```python
from build123d import *

# Parameters (mm, degrees)
SKETCH_1_R      = 50
EXTRUDE_1_DEPTH = 10


with BuildPart() as part:
    # ｽｹｯﾁ1 → ﾎﾞｽ - 押し出し1 (new body)
    with BuildSketch(Plane(origin=(0, 0, 0), x_dir=(1, 0, 0), z_dir=(0, 1, 0))):
        Circle(SKETCH_1_R)
        with BuildLine():
            Line((-3.420201433, 9.396926208), (-13.680805733, 37.587704831))
            ThreePointArc((-13.680805733, 37.587704831), (0, 40), (13.680805733, 37.587704831))
            Line((13.680805733, 37.587704831), (3.420201433, 9.396926208))
            ThreePointArc((3.420201433, 9.396926208), (0, 10), (-3.420201433, 9.396926208))
        make_face(mode=Mode.SUBTRACT)
        with BuildLine():
            Line((6.428376097, 7.661310457), (25.712004387, 30.64264375))
            ThreePointArc((25.712004387, 30.64264375), (34.641516151, 20.000866025), (39.39281012, 6.946793132))
            Line((39.39281012, 6.946793132), (9.84857753, 1.737347802))
            ThreePointArc((9.84857753, 1.737347802), (8.660754038, 5.000866025), (6.428376097, 7.661310457))
        make_face(mode=Mode.SUBTRACT)
        with BuildLine():
            Line((9.84957753, -1.735615751), (39.39381012, -6.945061081))
            ThreePointArc((39.39381012, -6.945061081), (34.642516151, -19.999133975), (25.713004387, -30.640911699))
            Line((25.713004387, -30.640911699), (6.429376097, -7.659578406))
            ThreePointArc((6.429376097, -7.659578406), (8.661754038, -4.999133975), (9.84957753, -1.735615751))
        make_face(mode=Mode.SUBTRACT)
        with BuildLine():
            Line((3.422201433, -9.396926208), (13.682805733, -37.587704831))
            ThreePointArc((13.682805733, -37.587704831), (0.002, -40), (-13.678805733, -37.587704831))
            Line((-13.678805733, -37.587704831), (-3.418201433, -9.396926208))
            ThreePointArc((-3.418201433, -9.396926208), (0.002, -10), (3.422201433, -9.396926208))
        make_face(mode=Mode.SUBTRACT)
        with BuildLine():
            Line((-6.426376097, -7.661310457), (-25.710004387, -30.64264375))
            ThreePointArc((-25.710004387, -30.64264375), (-34.639516151, -20.000866025), (-39.39081012, -6.946793132))
            Line((-39.39081012, -6.946793132), (-9.84657753, -1.737347802))
            ThreePointArc((-9.84657753, -1.737347802), (-8.658754038, -5.000866025), (-6.426376097, -7.661310457))
        make_face(mode=Mode.SUBTRACT)
        with BuildLine():
            Line((-9.84757753, 1.735615751), (-39.39181012, 6.945061081))
            ThreePointArc((-39.39181012, 6.945061081), (-34.640516151, 19.999133975), (-25.711004387, 30.640911699))
            Line((-25.711004387, 30.640911699), (-6.427376097, 7.659578406))
            ThreePointArc((-6.427376097, 7.659578406), (-8.659754038, 4.999133975), (-9.84757753, 1.735615751))
        make_face(mode=Mode.SUBTRACT)
    extrude(amount=EXTRUDE_1_DEPTH)


solid = part.part
```
Geometry check sheet. Reference: the model listing, model coordinates, mm. A direction names the side the tool comes from. Coordinates: 2 decimals unless noted, no trailing zeros. Order: outer loops, then holes, each group sorted by start corner. A loop starts at its lowest first (then second) coordinate and runs counter-clockwise, first axis right, second up. Notation, with made-up numbers: M -14,20 L -3,20 A22 ccw -3,36 Z; hole C 50.25,-22 d2. An arc over 180 degrees is marked long. One line per question, with ' | ' between items. Start each with the question number.
Item 1: Gauge pin test, flat ends, axial feed: pin 1 (6 mm diameter, centred on x = 18, y = 1.5, fed in from +Z); pin 2 (5 mm diameter, centred on y = 6, z = -25, fed in from -X). Record the tip position at first contact, or that the pin passes through.
Item 2: Draft check along X on faces 1 (the cylindrical face through (-34.738, 4.93, -19.83)), 2 (the cylindrical face through (47.69, 4.93, -15.02)), 3 (the flat face through (-1, 10, -1)). Enter one of: pulls with the +X half, pulls with the -X half, needs draft (parallel to the pull), parting line crosses it, or undercut.
Item 3: Cross-section at C-C on z = -22. Enter the section's corners in (x, y).
Item 4: Cross-section at A-A on y = 7.75. Enter the section's corners in (x, z).
Item 5: Cross-section at B-B on x = 34.5. Enter the section's corners in (y, z).
Item 6: Cross-section at D-D on z = -3. Enter the section's corners in (x, y).
Item 7: Set-up check for faces 4 (the flat face through (-1, 0, -1)), 5 (the flat face through (24.4, 4.9, 4.3)): record each of +Z, -Z, +X, -X, +Y, -Y from which the full face is reachable in a straight line by a thin tool's end or side.
Item 8: Material ranges on L1, parallel to Z at x = 17, y = 0.5; L2, parallel to X at y = 8.5, z = 12; L3, parallel to X at y = 1.25, z = 14, recorded low to high. Write a range as [from, to].
Findings:
1) pin 1: stops at z = 47.7 | pin 2: stops at x = -44.65
2) face 1: undercut | face 2: parting line crosses it | face 3: needs draft
3) outline: M -44.9,0 L -33.41,0 L -33.41,10 L -44.9,10 Z; M -18.46,0 L -8.01,0 L -8.01,10 L -18.46,10 Z; M 8.01,0 L 18.46,0 L 18.46,10 L 8.01,10 Z; M 33.41,0 L 44.9,0 L 44.9,10 L 33.41,10 Z
4) outline: C 0,0 d100; hole M -39.39,-6.95 A40 ccw -25.71,-30.64 L -6.43,-7.66 A10 cw -9.85,-1.74 Z; hole M -39.39,6.95 L -9.85,1.74 A10 cw -6.43,7.66 L -25.71,30.64 A40 ccw Z; hole M -13.68,-37.59 A40 ccw 13.68,-37.59 L 3.42,-9.4 A10 cw -3.42,-9.4 Z; hole M -13.68,37.59 L -3.42,9.4 A10 cw 3.42,9.4 L 13.68,37.59 A40 ccw Z; hole M 6.43,-7.66 L 25.71,-30.64 A40 ccw 39.39,-6.95 L 9.85,-1.74 A10 cw Z; hole M 6.43,7.66 A10 cw 9.85,1.74 L 39.39,6.95 A40 ccw 25.71,30.64 Z
5) outline: M 0,-36.19 L 10,-36.19 L 10,-20.24 L 0,-20.24 Z; M 0,-6.08 L 10,-6.08 L 10,6.08 L 0,6.08 Z; M 0,20.24 L 10,20.24 L 10,36.19 L 0,36.19 Z
6) outline: M -49.91,0 L -17.02,0 L -17.02,10 L -49.91,10 Z; M -9.54,0 L 9.54,0 L 9.54,10 L -9.54,10 Z; M 17.01,0 L 49.91,0 L 49.91,10 L 17.01,10 Z
7) face 4: +Z, -Z, +X, -X, -Y | face 5: +Y, -Y
8) L1: z = [-47.02, -20.26], [-3, 3], [20.26, 47.02] | L2: x = [-48.54, -38.16], [-10.07, -4.37], [4.37, 10.07], [38.16, 48.54] | L3: x = [-48, -37.47], [-11.75, -5.09], [5.1, 11.75], [37.47, 48]
